CAD build for the part. Positions are in the model's coordinates, mm. A direction names the side the tool comes from. Give positions to 0.01 mm unless a question says otherwise; leave off trailing zeros. Loops run counter-clockwise (first coordinate to the right, second up) from the corner with the lowest first, then second, coordinate; pieces in that order, holes last. Notation, with made-up numbers: (41, 40.5) - (84, 40.5) arc R22 cw to (84, 69.5) - close; hole circle Ø8 at (49, 74.5). An arc over 180 degrees is marked (long way). Return JSON: item names as keys, results as strings.
from build123d import *

# Parameters (mm, degrees)
SKETCH1_W           = 30
SKETCH1_H           = 30
BOSS_EXTRUDE1_DEPTH = 10
SKETCH3_W           = 55
SKETCH3_H           = 30
SKETCH3_W_2         = 30
BOSS_EXTRUDE3_DEPTH = 10


with BuildPart() as part:
    # Sketch1 → Boss-Extrude1 (new body)
    with BuildSketch(Plane(origin=(0, 0, 0), x_dir=(1, 0, 0), z_dir=(0, 1, 0))):
        Rectangle(SKETCH1_W, SKETCH1_H)
    extrude(amount=BOSS_EXTRUDE1_DEPTH)

    # Sketch3 → Boss-Extrude3 (add)
    with BuildSketch(Plane.XZ):
        with Locations((42.5, 0)):
            Rectangle(SKETCH3_W, SKETCH3_H)
        Polygon((-15, -15), (-15, -100), (70, -15), (15, -15), align=None)
        Rectangle(SKETCH3_W_2, SKETCH3_H)
    extrude(amount=BOSS_EXTRUDE3_DEPTH)


solid = part.part
1. Drop flat-ended pins along their axis: P1, Ø3, axis at x = -1.5, y = 3, coming from the -Z side; P2, Ø4, axis at x = 22, z = -62.5, coming from the +Y side; P3, Ø3, axis at y = 3.5, z = 4.5, coming from the +X side. Give the stop position or say it passes through.
Values follow:
{"P1": "stops at z = -15", "P2": "stops at y = 0", "P3": "stops at x = 15"}
2. Which spindle directions (+Z, -Z, +X, -X, +Y, -Y) get a long thin tool onto all of the face, cutting with end or side? Do faces 1 (the face through (15, 5, 0)), 2 (the face through (27, -5, -58)), 3 (the face through (0, 5, -15)). Say none if no direction does.
Values follow:
{"face 1": "+Z, -Z, +X, +Y", "face 2": "-Z, +X, +Y, -Y", "face 3": "-Z, +X, -X, +Y"}
3. Cut at B-B, the plane x = 55. Write the cut outline in (y, z).
Values follow:
{"outline": "(-10, -30) - (0, -30) - (0, 15) - (-10, 15) - close"}
4. Cut at C-C, the plane z = 4. Write the cut outline in (x, y).
Values follow:
{"outline": "(-15, -10) - (70, -10) - (70, 0) - (15, 0) - (15, 10) - (-15, 10) - close"}
5. Drill centre lines: probe 1 along Y at (x, z) = (56.5, -15); probe 2 along Z at (x, y) = (5, 7.5). Where is each one in solid material? Low to high.
Values follow:
{"probe 1": "y = -10 to 0", "probe 2": "z = -15 to 15"}
6. Cut at D-D, the plane x = -2. Write the cut outline in (y, z).
Values follow:
{"outline": "(-10, -87) - (0, -87) - (0, -15) - (10, -15) - (10, 15) - (-10, 15) - close"}
7. Cut at A-A, the plane z = -44.5. Write the cut outline in (x, y).
Values follow:
{"outline": "(-15, -10) - (40.5, -10) - (40.5, 0) - (-15, 0) - close"}
